```python
from build123d import *

# Parameters (mm, degrees)
F0_W     = 25.94131
F0_H     = 35.997212
F1_DEPTH = 11.938
F2_W     = 30.896392
F2_H     = 44.304264
F3_DEPTH = 1.27
F4_W     = 30.896392
F4_H     = 44.304264
F5_DEPTH = 1.524
F6_R     = 5.08


with BuildPart() as f1:
    # F0 (on Top) → F1 (new body)
    with BuildSketch(Plane.XY):
        with Locations((-0.437213, -17.998606)):
            Rectangle(F0_W, F0_H)
    extrude(amount=F1_DEPTH)

    # F2 (on face) → F3 (join)
    with BuildSketch(Plane.XY.offset(11.938)):
        with Locations((-0.58295, -18.508689)):
            Rectangle(F2_W, F2_H)
    extrude(amount=F3_DEPTH)

    # F4 (on face) → F5 (join)
    with BuildSketch(Plane(origin=(0, 0, 0), x_dir=(1, 0, 0), z_dir=(0, 0, -1))):
        with Locations((-0.58295, 18.508689)):
            Rectangle(F4_W, F4_H)
    extrude(amount=F5_DEPTH)

    # F6
    f6_edges = [f1.edges().sort_by_distance(p)[0] for p in [
        (14.865246, -40.660821, -0.762),
        (14.865246, -40.660821, 12.573),
        (14.865246, 3.643443, -0.762),
        (-16.031146, -40.660821, -0.762),
        (-16.031146, -40.660821, 12.573),
        (14.865246, 3.643443, 12.573),
        (-16.031146, 3.643443, 12.573),
        (-16.031146, 3.643443, -0.762),
    ]]
    fillet(f6_edges, radius=F6_R)


solid = f1.part
```
Here's how the part is built. I have some questions about the finished solid (model axes, mm). A direction names the side the tool comes from. Give positions to 0.01 mm unless a question says otherwise; leave off trailing zeros. Write each loop counter-clockwise with the first axis right and the second up, starting at its lowest first coordinate (ties: lowest second). Pieces come first, ordered by that corner, then holes. Notation, with made-up numbers: M -11,4.25 L 16,4.25 A16 ccw 16,27.25 Z; hole C 42.5,35 d1. An arc over 180 degrees is marked long. Put each result on its own line as item: value. Start each with the question number.
Item 1: If we section it at D-D, the plane z = 11.25: Write out the boundary of the cut face in (x, y), then the cut area to 3 significant figures.
Item 2: Thinking about a two-plate mould opening in Z: for faces 4 (the flat face through (-1, -18, 13.208)), 5 (the flat face through (-1, -19, -1.524)), 6 (the cylindrical face through (-14.6, 2.1, -0.8)), 7 (the flat face through (12.533, -18, 6)), which applies, +Z half, -Z half, draft (parallel to the pull), parting line (faces both ways), or undercut?
Item 3: If we section it at C-C, the plane y = -37: Write out the boundary of the cut face in (x, z).
Item 4: Will these pins go through, and if not, where does the flat tip stop? pin 1 (6 mm diameter, centred on x = 3.5, z = 7.5, fed in from +Y); pin 2 (3.5 mm diameter, centred on y = -21, z = 8, fed in from +X); pin 3 (6 mm diameter, centred on x = 3.5, z = 6, fed in from -Y).
Item 5: If we section it at A-A, the plane y = -4: Write out the boundary of the cut face in (x, z), then the cut area to 3 significant figures.
Item 6: If we section it at B-B, the plane x = -2: Write out the boundary of the cut face in (y, z), then the cut area to 3 significant figures.
Item 7: I need wall thicknesses on L1, parallel to Y at x = -7, z = 11; L2, parallel to Z at x = 6.5, y = 1; L3, parallel to X at y = -7, z = 11. Which ranges of each line are inside material? Lowest first, please. Write a range as from..to.
Item 8: On a 3-axis mill with a long thin cutter (end or side, diameter ignored), from which of +Z, -Z, +X, -X, +Y, -Y can I reach the whole of each face in a straight line? I mean faces 1 (the flat face through (-13.408, -18, 6)), 2 (the flat face through (13, -18, 11.938)), 3 (the flat face through (-1, -40.661, -1)). Say none if no direction works.
Values:
1. outline: M -13.41,-36 L 12.53,-36 L 12.53,0 L -13.41,0 Z
1. area: 934 mm²
2. face 4: +Z half
2. face 5: -Z half
2. face 6: draft
2. face 7: undercut
3. outline: M -15.83,-1.52 L 14.66,-1.52 L 14.66,0 L -15.83,0 Z; M -15.83,11.94 L 14.66,11.94 L 14.66,13.21 L -15.83,13.21 Z
4. pin 1: y = 0
4. pin 2: x = 12.53
4. pin 3: y = -36
5. outline: M -16.03,-1.52 L 14.87,-1.52 L 14.87,0 L 12.53,0 L 12.53,11.94 L 14.87,11.94 L 14.87,13.21 L -16.03,13.21 L -16.03,11.94 L -13.41,11.94 L -13.41,0 L -16.03,0 Z
5. area: 396 mm²
6. outline: M -40.66,-1.52 L 3.64,-1.52 L 3.64,0 L 0,0 L 0,11.94 L 3.64,11.94 L 3.64,13.21 L -40.66,13.21 L -40.66,11.94 L -36,11.94 L -36,0 L -40.66,0 Z
6. area: 554 mm²
7. L1: -36..0
7. L2: -1.52..0, 11.94..13.21
7. L3: -13.41..12.53
8. face 1: -X, +Y, -Y
8. face 2: none
8. face 3: +Z, -Z, +X, -X, -Y
